from build123d import *

# Parameters (mm, degrees)
SKETCH11_W         = 135.340286593
SKETCH11_H         = 57.113739626
CUT_EXTRUDE1_DEPTH = 18.6646359


with BuildPart() as part:
    # Sweep-Thin1: sweep along a path in Sketch2
    with BuildLine(Plane(origin=(0, 0, 0), x_dir=(1, 0, 0), z_dir=(0, 1, 0))) as sweep_thin1_path:
        Line((439.99296617, 259.17166973), (431.5, 250))
        Line((431.5, 250), (200, 0))
        Line((200, 0), (0, 0))
        Line((0, 0), (-250, 0))
        Line((-250, 0), (-250, 125))
        Line((-250, 125), (0, 125))
        Line((0, 125), (0, 250))
    # Sketch6 → Sweep-Thin1 (sweep)
    with BuildSketch(Plane.XY.offset(-250)):
        with BuildLine():
            Line((4.5, 12.5), (-4.5, 12.5))
            ThreePointArc((-4.5, 12.5), (-10.156854249, 10.156854249), (-12.5, 4.5))
            Line((-12.5, 4.5), (-12.5, -4.5))
            ThreePointArc((-12.5, -4.5), (-10.156854249, -10.156854249), (-4.5, -12.5))
            Line((-4.5, -12.5), (4.5, -12.5))
            ThreePointArc((4.5, -12.5), (10.156854249, -10.156854249), (12.5, -4.5))
            Line((12.5, -4.5), (12.5, 4.5))
            ThreePointArc((12.5, 4.5), (10.156854249, 10.156854249), (4.5, 12.5))
        make_face()
        with BuildLine():
            Line((4.5, 9.5), (-4.5, 9.5))
            ThreePointArc((-4.5, 9.5), (-8.035533906, 8.035533906), (-9.5, 4.5))
            Line((-9.5, 4.5), (-9.5, -4.5))
            ThreePointArc((-9.5, -4.5), (-8.035533906, -8.035533906), (-4.5, -9.5))
            Line((-4.5, -9.5), (4.5, -9.5))
            ThreePointArc((4.5, -9.5), (8.035533906, -8.035533906), (9.5, -4.5))
            Line((9.5, -4.5), (9.5, 4.5))
            ThreePointArc((9.5, 4.5), (8.035533906, 8.035533906), (4.5, 9.5))
        make_face(mode=Mode.SUBTRACT)
    sweep(path=sweep_thin1_path.line, transition=Transition.RIGHT)

    # Sketch11 → Cut-Extrude1 (cut, through all)
    with BuildSketch(Plane.XY.offset(-250)):
        with Locations((387.319769347, 0)):
            Rectangle(SKETCH11_W, SKETCH11_H)
    extrude(amount=-CUT_EXTRUDE1_DEPTH, mode=Mode.SUBTRACT)


solid = part.part
Can you work these out from the model? Positions are in its coordinate system, mm. A direction names the side the tool comes from. Give positions to 0.01 mm unless a question says otherwise; leave off trailing zeros. Order: outer loops, then holes, each group sorted by start corner. A loop starts at its lowest first (then second) coordinate and runs counter-clockwise, first axis right, second up. Notation, with made-up numbers: M 18,-22.5 L 57,-22.5 A8 ccw 57,-16.5 Z; hole C -8,-16.5 d4. An arc over 180 degrees is marked long. Use one line per item in the form item = value.
Item 1: Will these pins go through, and if not, where does the flat tip stop? pin 1 Ø7 at (x, y) = (-174, -0.5) entering from -Z; pin 2 Ø4.5 at (y, z) = (1.5, -216.5) entering from -X; pin 3 Ø10 at (y, z) = (1, -195.5) entering from +X.
Values follow:
pin_1 = -137.5
pin_2 = -12.5
pin_3 = 402.7
Item 2: If I drill on line 1 along Z through (x, y) = (-26, -5); line 2 along X through (y, z) = (-6.5, -37); line 3 along X through (y, z) = (-8.5, -122.5), over which ranges is the centre line in solid material (lowest first)? Write a range as [from, to].
Values follow:
line_1 = [-137.48, -134.47], [-115.53, -112.52], [-12.48, -9.47], [9.47, 12.48]
line_2 = [-262.25, -259.08], [-240.92, -237.75], [217.57, 221.88], [246.64, 250.95]
line_3 = [-261.43, -257.5], [7.5, 11.43], [297.86, 303.21], [323.66, 329.01]
Item 3: Thinking about a two-plate mould opening in Z: for faces 1 (the flat face through (112, 9.5, -2)), 2 (the flat face through (431, -11, -250)), 3 (the flat face through (0, 12.5, -139)), which applies, pulls with the +Z half, pulls with the -Z half, needs draft (parallel to the pull), parting line crosses it, or undercut?
Values follow:
face_1 = undercut
face_2 = pulls with the -Z half
face_3 = needs draft
Item 4: If we section it at A-A, the plane x = -200.5: Count the separate pieces of the cut face and the enclosed holes in it, and give its area (3 significant figures).
Values follow:
separate_pieces = 2
enclosed_holes = 2
area = 461 mm^2
Item 5: For faces 4 (the flat face through (-11, 0, -250)), 5 (the flat face through (305.642, 0.063, -128.066)), 6 (the cylindrical face through (306.004, 10.219, -129.332)), 7 (the cylindrical face through (305.91, -10.09, -129.42)), 8 (the flat face through (302.962, -0.063, -129.587)), which set-ups out of +Z, -Z, +X, -X, +Y, -Y let a thin tool reach every point of the face, with its end or its side?
Values follow:
face_4 = -Z, +X, -X, +Y, -Y
face_5 = none
face_6 = -Z, +Y
face_7 = -Z, -Y
face_8 = -Z, +Y, -Y
Item 6: If we section it at B-B, the plane x = 104.5: Write out the boundary of the cut face in (y, z).
Values follow:
outline = M -12.5,-4.5 A8 ccw -4.5,-12.5 L 4.5,-12.5 A8 ccw 12.5,-4.5 L 12.5,4.5 A8 ccw 4.5,12.5 L -4.5,12.5 A8 ccw -12.5,4.5 Z; hole M -9.5,-4.5 A5 ccw -4.5,-9.5 L 4.5,-9.5 A5 ccw 9.5,-4.5 L 9.5,4.5 A5 ccw 4.5,9.5 L -4.5,9.5 A5 ccw -9.5,4.5 Z
